```python
from build123d import *

# Parameters (mm, degrees)
F2_DEPTH    = 4
F3_C1_SIZE  = 2
F3_C2_SIZE  = 2
F3_C3_SIZE  = 2
F3_C4_SIZE  = 2
F3_C5_SIZE  = 2
F3_C6_SIZE  = 2
F3_C7_SIZE  = 2
F3_C8_SIZE  = 2
F3_C9_SIZE  = 2
F3_C10_SIZE = 2


with BuildPart() as f2:
    # F1 (on Top) → F2 (new body)
    with BuildSketch(Plane.XY):
        Polygon((-25, 0), (0, 0), (-2.0441389628, 6.2647895141), (-25, 5.3083011104), align=None)
        Polygon((-25, 5.3083011104), (-2.0441389628, 6.2647895141), (-4.0478985191, 12.4058259531), (-75.8, 6.4056137967), (-75.8, 3.1916472924), (-51.2, 4.2166410704), (-51.2, 7.6929950155), (-50.4, 7.6929950155), (-50.4, 4.2499742014), (-25.8, 5.2749679794), (-25.8, 7.6929950155), (-25, 7.6929950155), align=None)
        Polygon((-50.4, 0), (-25.8, 0), (-25.8, 5.2749679794), (-50.4, 4.2499742014), align=None)
        Polygon((-75.8, 0), (-51.2, 0), (-51.2, 4.2166410704), (-75.8, 3.1916472924), align=None)
        Polygon((-51.2, 4.2166410704), (-50.4, 4.2499742014), (-50.4, 7.6929950155), (-51.2, 7.6929950155), align=None)
        Polygon((-25.8, 5.2749679794), (-25, 5.3083011104), (-25, 7.6929950155), (-25.8, 7.6929950155), align=None)
        Polygon((-76.6, 3.1583141614), (-76.6, 6.3387144359), (-101.2, 4.2815590912), (-101.2, 2.1333203834), align=None)
        Polygon((-75.8, 3.1916472924), (-75.8, 6.4056137967), (-76.6, 6.3387144359), (-76.6, 3.1583141614), align=None)
        Polygon((-76.6, 0), (-76.6, 3.1583141614), (-101.2, 2.1333203834), (-101.2, 0), align=None)
        Polygon((-101.2, 2.1333203834), (-101.2, 4.2815590912), (-102, 4.2146597304), (-102, 2.0999872524), align=None)
        Polygon((-102, 0), (-102, 2.0999872524), (-126.6, 1.0749934745), (-126.6, 0), align=None)
        Polygon((-102, 2.0999872524), (-102, 4.2146597304), (-126.6, 2.1575043858), (-126.6, 1.0749934745), align=None)
        Polygon((-126.6, 1.0749934745), (-126.6, 2.1575043858), (-127.4, 2.090605025), (-127.4, 1.0416603435), align=None)
        Polygon((-127.4, 1.0416603435), (-127.4, 2.090605025), (-152.4, 0), align=None)
        Polygon((-127.4, 1.0416603435), (-152.4, 0), (-127.4, 0), align=None)
    extrude(amount=F2_DEPTH)

    # F3: chamfer of 2 on 11 edges, made by hand

    # F3_c1
    f3_c1_edges = [f2.edges().sort_by_distance(p)[0] for p in [
        (-12.5, 0, 4),
    ]]
    chamfer(f3_c1_edges, length=F3_C1_SIZE)

    # F3_c2
    f3_c2_edges = [f2.edges().sort_by_distance(p)[0] for p in [
        (-2.350239386, 7.2029129766, 4),
    ]]
    chamfer(f3_c2_edges, length=F3_C2_SIZE)

    # F3_c3
    f3_c3_edges = [f2.edges().sort_by_distance(p)[0] for p in [
        (-139.9, 0, 4),
    ]]
    chamfer(f3_c3_edges, length=F3_C3_SIZE)

    # F3_c4
    f3_c4_edges = [f2.edges().sort_by_distance(p)[0] for p in [
        (-101.6, 2.1166538179, 4),
    ]]
    chamfer(f3_c4_edges, length=F3_C4_SIZE)

    # F3_c5
    f3_c5_edges = [f2.edges().sort_by_distance(p)[0] for p in [
        (-88.9, 0, 4),
    ]]
    chamfer(f3_c5_edges, length=F3_C5_SIZE)

    # F3_c6
    f3_c6_edges = [f2.edges().sort_by_distance(p)[0] for p in [
        (-76.2, 3.1749807269, 4),
    ]]
    chamfer(f3_c6_edges, length=F3_C6_SIZE)

    # F3_c7
    f3_c7_edges = [f2.edges().sort_by_distance(p)[0] for p in [
        (-63.5, 0, 4),
    ]]
    chamfer(f3_c7_edges, length=F3_C7_SIZE)

    # F3_c8
    f3_c8_edges = [f2.edges().sort_by_distance(p)[0] for p in [
        (-50.8, 4.2333076359, 4),
    ]]
    chamfer(f3_c8_edges, length=F3_C8_SIZE)

    # F3_c9
    f3_c9_edges = [f2.edges().sort_by_distance(p)[0] for p in [
        (-38.1, 0, 4),
    ]]
    chamfer(f3_c9_edges, length=F3_C9_SIZE)

    # F3_c10
    f3_c10_edges = [f2.edges().sort_by_distance(p)[0] for p in [
        (-25.4, 5.2916345449, 4),
    ]]
    chamfer(f3_c10_edges, length=F3_C10_SIZE)

    # F4: F2 across face


with BuildPart() as f2_1:
    add(f2.part)
    add(f2.part.mirror(Plane(origin=(-75.6988371999, 6.414073455, 1.938990945), x_dir=(-0.9965217286, -0.0833333333, 0), z_dir=(-0.0833333333, 0.9965217286, 0))))


solid = f2_1.part
```
Work out the finished part from the listing and answer in its coordinate system (mm). A direction names the side the tool comes from. Give positions to 0.01 mm unless a question says otherwise; leave off trailing zeros. Loops run counter-clockwise (first coordinate to the right, second up) from the corner with the lowest first, then second, coordinate; pieces in that order, holes last. Notation, with made-up numbers: (46, -17.5) -> (61, -17.5) arc R12 cw to (61, 3.5) -> close; hole circle Ø1 at (73, -9). An arc over 180 degrees is marked (long way). One line per question, with ' | ' between items. Start each with the question number.
1) Section B-B, the plane x = -17 is taken. Determine the outline of the cut face in (y, z), then the cut area to 3 significant figures.
2) For faces 1 (the face through (-102.44, 6.83, 1.97)), 2 (the face through (-101.2, 1.6, 2)), 3 (the face through (-26.29, 18.31, 1.97)), determine the directions among +Z, -Z, +X, -X, +Y, -Y from which every point of the face is accessible in a straight line to the end or side of a thin tool.
3) Section A-A, the plane x = -62.5 is taken. Determine the outline of the cut face in (y, z).
4) Determine the mould class of faces 4 (the face through (-51.406, 14.5, 1.972)), 5 (the face through (-75.8, 2, 2)), 6 (the face through (-89.788, 9.546, 2.986)) for opening direction Y: +Y half, -Y half, draft (parallel to the pull), parting line (faces both ways), or undercut.
5) Each of these flat-tipped pins is pushed along its axis until it touches: pin 1 (0.5 mm diameter, centred on y = 0.5, z = 1.5, fed in from +X); pin 2 (2 mm diameter, centred on y = 1.5, z = 1.5, fed in from +X); pin 3 (1.5 mm diameter, centred on x = -22, y = 15.5, fed in from -Z); pin 4 (2 mm diameter, centred on y = 10.5, z = 0.5, fed in from +X). Where does it stop, or does it pass through?
6) Straight lines are drawn through the part: L1, parallel to Y at x = -128, z = 0.9; L2, parallel to Y at x = -119, z = 1.4; L3, parallel to Z at x = -11, y = 1.75. For each, find the intervals that lie inside material, in ascending order.
Resolved:
1) outline: (0, 0) -> (22.8, 0) -> (22.8, 2) -> (20.78, 4) -> (2, 4) -> (0, 2) -> close | area: 87.2 mm2
2) face 1: +Z, +Y | face 2: +Z, -Y | face 3: +Z
3) outline: (0, 0) -> (15.14, 0) -> (15.14, 2) -> (13.11, 4) -> (2, 4) -> (0, 2) -> close
4) face 4: undercut | face 5: draft | face 6: +Y half
5) pin 1: x = -0.08 | pin 2: x = -0.16 | pin 3: z = 0 | pin 4: x = -3.1
6) L1: 0 to 4.11 | L2: 0 to 5.63 | L3: 0 to 3.75
